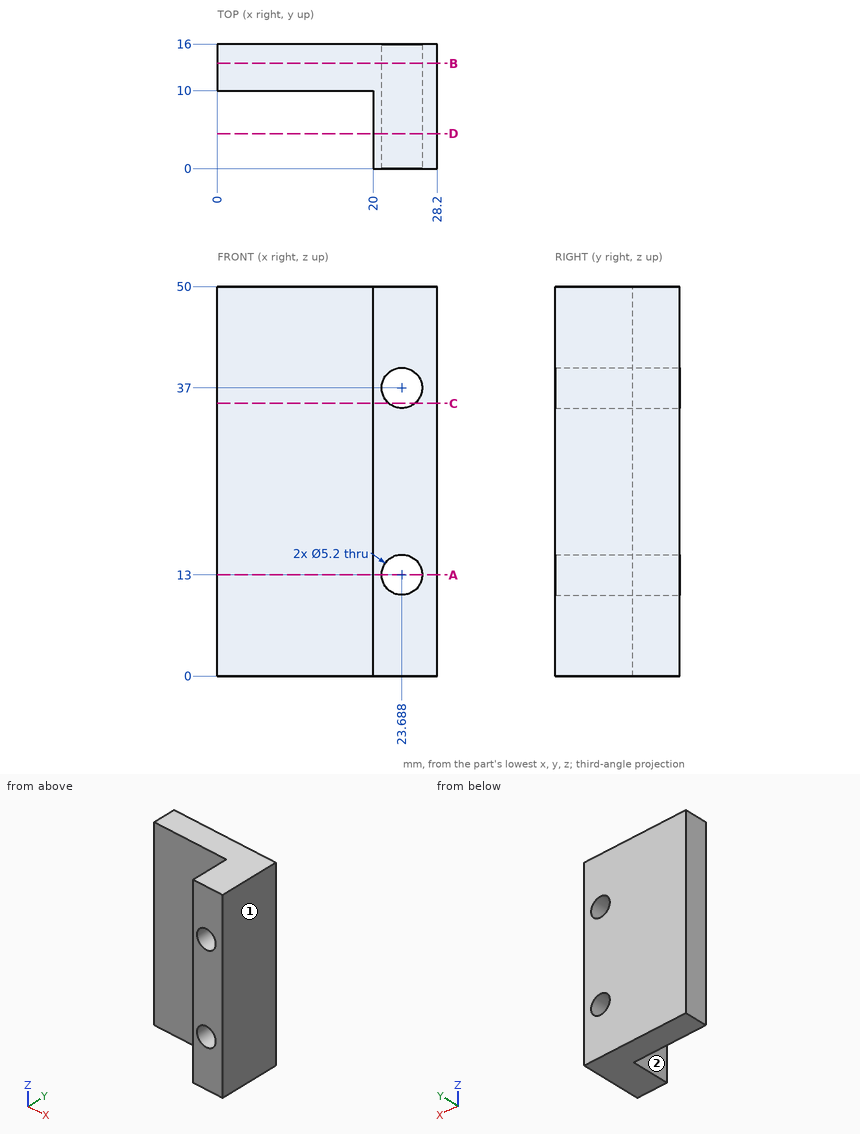
Source: three-view drawing plus pictorial views. Frame: mm from the lowest corner of the part. A direction names the side the tool comes from. Give positions to 0.01 mm unless a question says otherwise; leave off trailing zeros. Loops run counter-clockwise (first coordinate to the right, second up) from the corner with the lowest first, then second, coordinate; pieces in that order, holes last. Notation, with made-up numbers: (-8, -16.75) -> (20, -16.75) arc R14 ccw to (20, -12.75) -> close; hole circle Ø6 at (65, 15). An arc over 180 degrees is marked (long way). Use a Markdown table: item, result. Add a question column.
(1) Access query for the marked faces 1 and 2. Directions: +Z, -Z, +X, -X, +Y, -Y. A direction counts if a zero-diameter tool reaches every point of the face in a straight line with its end or side. Return the directions, or none.
(2) Section query A-A (z = 13). Output: boundary loops of the cut face in (x, y), then the cut area to 3 significant figures.
(3) Section query D-D (y = 4.5). Output: boundary loops of the cut face in (x, z).
(4) First-contact query: pin 1 Ø12 at (x, z) = (11.5, 6.5) entering from -Y; pin 2 Ø4 at (x, y) = (14, 7) entering from -Z. Flat tips, straight axial feed; report the tip coordinate or a pass-through.
(5) Ray query, line 1 (Z direction, x = 22.75, y = 8.5) (1 decimal); line 2 (X direction, y = 9.75, z = 13); line 3 (X direction, y = 10.5, z = 37). Return the intervals inside material, ascending.
(6) Section query C-C (z = 35). Output: boundary loops of the cut face in (x, y).
(7) Section query B-B (y = 13.5). Output: boundary loops of the cut face in (x, z).
Checked values:
| question | item | result |
|---|---|---|
| 1 | face 1 | +Z, -Z, +X, +Y, -Y |
| 1 | face 2 | +Z, -Z, -X, -Y |
| 2 | outline | (0, 10) -> (20, 10) -> (20, 0) -> (21.09, 0) -> (21.09, 16) -> (0, 16) -> close; (26.29, 0) -> (28.2, 0) -> (28.2, 16) -> (26.29, 16) -> close |
| 2 | area | 168 mm^2 |
| 3 | outline | (20, 0) -> (28.2, 0) -> (28.2, 50) -> (20, 50) -> close; hole circle Ø5.2 at (23.69, 13); hole circle Ø5.2 at (23.69, 37) |
| 4 | pin 1 | y = 10 |
| 4 | pin 2 | through |
| 5 | line 1 | 0 to 10.6, 15.4 to 34.6, 39.4 to 50 |
| 5 | line 2 | 20 to 21.09, 26.29 to 28.2 |
| 5 | line 3 | 0 to 21.09, 26.29 to 28.2 |
| 6 | outline | (0, 10) -> (20, 10) -> (20, 0) -> (22.03, 0) -> (22.03, 16) -> (0, 16) -> close; (25.35, 0) -> (28.2, 0) -> (28.2, 16) -> (25.35, 16) -> close |
| 7 | outline | (0, 0) -> (28.2, 0) -> (28.2, 50) -> (0, 50) -> close; hole circle Ø5.2 at (23.69, 13); hole circle Ø5.2 at (23.69, 37) |
